```python
from build123d import *

# Parameters (mm, degrees)
SKETCH3_W              = 411.1625
SKETCH3_H              = 277.368
BOSS_EXTRUDE1_DEPTH    = 1.5875
CUT_EXTRUDE1_DEPTH     = 25.4
F_10_CLEARANCE_HOLE1_D = 4.9784
F_10_CLEARANCE_HOLE2_D = 4.9784
F_10_CLEARANCE_HOLE3_D = 4.9784
F_10_CLEARANCE_HOLE4_D = 4.9784
F_10_CLEARANCE_HOLE5_D = 4.9784


with BuildPart() as part:
    # Sketch3 → Boss-Extrude1 (new, symmetric)
    with BuildSketch(Plane.XY):
        Rectangle(SKETCH3_W, SKETCH3_H)
    extrude(amount=BOSS_EXTRUDE1_DEPTH, both=True)

    # Sketch4 → Cut-Extrude1 (cut)
    with BuildSketch(Plane.XY.offset(1.5875)):
        with BuildLine():
            Line((-8.89, 98.4326708), (8.89, 98.4326708))
            ThreePointArc((8.89, 98.4326708), (12.482102448, 96.944773248), (13.97, 93.3526708))
            Line((13.97, 93.3526708), (13.97, 52.7126708))
            ThreePointArc((13.97, 52.7126708), (12.482102448, 49.120568352), (8.89, 47.6326708))
            Line((8.89, 47.6326708), (-8.89, 47.6326708))
            ThreePointArc((-8.89, 47.6326708), (-12.482102448, 49.120568352), (-13.97, 52.7126708))
            Line((-13.97, 52.7126708), (-13.97, 93.3526708))
            ThreePointArc((-13.97, 93.3526708), (-12.482102448, 96.944773248), (-8.89, 98.4326708))
        make_face()
        with BuildLine():
            Line((67.31, 98.4326708), (85.09, 98.4326708))
            ThreePointArc((85.09, 98.4326708), (88.682102448, 96.944773248), (90.17, 93.3526708))
            Line((90.17, 93.3526708), (90.17, 52.7126708))
            ThreePointArc((90.17, 52.7126708), (88.682102448, 49.120568352), (85.09, 47.6326708))
            Line((85.09, 47.6326708), (67.31, 47.6326708))
            ThreePointArc((67.31, 47.6326708), (63.717897552, 49.120568352), (62.23, 52.7126708))
            Line((62.23, 52.7126708), (62.23, 93.3526708))
            ThreePointArc((62.23, 93.3526708), (63.717897552, 96.944773248), (67.31, 98.4326708))
        make_face()
        with BuildLine():
            Line((143.51, 98.4326708), (161.29, 98.4326708))
            ThreePointArc((161.29, 98.4326708), (164.882102448, 96.944773248), (166.37, 93.3526708))
            Line((166.37, 93.3526708), (166.37, 52.7126708))
            ThreePointArc((166.37, 52.7126708), (164.882102448, 49.120568352), (161.29, 47.6326708))
            Line((161.29, 47.6326708), (143.51, 47.6326708))
            ThreePointArc((143.51, 47.6326708), (139.917897552, 49.120568352), (138.43, 52.7126708))
            Line((138.43, 52.7126708), (138.43, 93.3526708))
            ThreePointArc((138.43, 93.3526708), (139.917897552, 96.944773248), (143.51, 98.4326708))
        make_face()
        with BuildLine():
            Line((-85.09, 98.4326708), (-67.31, 98.4326708))
            ThreePointArc((-67.31, 98.4326708), (-63.717897552, 96.944773248), (-62.23, 93.3526708))
            Line((-62.23, 93.3526708), (-62.23, 52.7126708))
            ThreePointArc((-62.23, 52.7126708), (-63.717897552, 49.120568352), (-67.31, 47.6326708))
            Line((-67.31, 47.6326708), (-85.09, 47.6326708))
            ThreePointArc((-85.09, 47.6326708), (-88.682102448, 49.120568352), (-90.17, 52.7126708))
            Line((-90.17, 52.7126708), (-90.17, 93.3526708))
            ThreePointArc((-90.17, 93.3526708), (-88.682102448, 96.944773248), (-85.09, 98.4326708))
        make_face()
        with BuildLine():
            Line((-161.29, 97.1626708), (-146.05, 97.1626708))
            ThreePointArc((-146.05, 97.1626708), (-142.457897552, 95.674773248), (-140.97, 92.0826708))
            Line((-140.97, 92.0826708), (-140.97, 53.9826708))
            ThreePointArc((-140.97, 53.9826708), (-142.457897552, 50.390568352), (-146.05, 48.9026708))
            Line((-146.05, 48.9026708), (-161.29, 48.9026708))
            ThreePointArc((-161.29, 48.9026708), (-164.882102448, 50.390568352), (-166.37, 53.9826708))
            Line((-166.37, 53.9826708), (-166.37, 92.0826708))
            ThreePointArc((-166.37, 92.0826708), (-164.882102448, 95.674773248), (-161.29, 97.1626708))
        make_face()
    extrude(amount=-CUT_EXTRUDE1_DEPTH, mode=Mode.SUBTRACT)

    # #10 Clearance Hole1 (through all)
    with Locations(Plane.XY.offset(1.5875)):
        with Locations((192.88125, 125.984), (-192.88125, -125.984), (192.88125, -125.984), (-192.88125, 125.984), (-192.88125, 0), (192.88125, 0)):
            Hole(F_10_CLEARANCE_HOLE1_D / 2)

    # #10 Clearance Hole2 (through all)
    with Locations(Plane.XY.offset(1.5875)):
        with Locations((0, -117.532545274)):
            Hole(F_10_CLEARANCE_HOLE2_D / 2)

    # #10 Clearance Hole3 (through all)
    with Locations(Plane.XY.offset(1.5875)):
        with Locations((-195.30625, -70.615668917)):
            Hole(F_10_CLEARANCE_HOLE3_D / 2)

    # #10 Clearance Hole4 (through all)
    with Locations(Plane.XY.offset(1.5875)):
        with Locations((-195.30625, -96.015668917)):
            Hole(F_10_CLEARANCE_HOLE4_D / 2)

    # #10 Clearance Hole5 (through all)
    with Locations(Plane.XY.offset(1.5875)):
        with Locations((195.30625, -68.024189157), (195.30625, -93.424189157)):
            Hole(F_10_CLEARANCE_HOLE5_D / 2)


solid = part.part
```
Read the model definition and answer for the solid it produces. Units are mm, in the model's axes. Give positions to 0.01 mm unless a question says otherwise; leave off trailing zeros. Write each loop counter-clockwise with the first axis right and the second up, starting at its lowest first coordinate (ties: lowest second). Pieces come first, ordered by that corner, then holes. Notation, with made-up numbers: M 72.5,42 L 111.5,42 A8 cw 111.5,48 Z; hole C -12.5,87 d8. An arc over 180 degrees is marked long. Put each result on its own line as item: value. Start each with the question number.
1. The part is cut by section B-B, the plane z = 1. Give the number of separate pieces and of enclosed holes in the cut face, and give its area (3 significant figures).
2. This flat-tipped pin is pushed along its axis until it touches: pin 1 Ø3 at (x, y) = (0, -117.53) entering from +Z. Where does it stop, or does it pass through?
3. Consider line 1 along Y through (x, z) = (0, 0.3); line 2 along Y through (x, z) = (6.5, -0.15); line 3 along X through (y, z) = (88, -0.6). Determine where each line is inside the solid, lowest interval first.
4. The part is cut by section A-A, the plane y = 58.5. Give the vertices of the cut face in (x, z).
Final values:
1. separate pieces: 1
1. enclosed holes: 16
1. area: 107,000 mm²
2. pin 1: passes through
3. line 1: y = -138.68 to -120.02, -115.04 to 47.63, 98.43 to 138.68
3. line 2: y = -138.68 to 47.63, 98.43 to 138.68
3. line 3: x = -205.58 to -166.37, -140.97 to -90.17, -62.23 to -13.97, 13.97 to 62.23, 90.17 to 138.43, 166.37 to 205.58
4. outline: M -205.58,-1.59 L -166.37,-1.59 L -166.37,1.59 L -205.58,1.59 Z; M -140.97,-1.59 L -90.17,-1.59 L -90.17,1.59 L -140.97,1.59 Z; M -62.23,-1.59 L -13.97,-1.59 L -13.97,1.59 L -62.23,1.59 Z; M 13.97,-1.59 L 62.23,-1.59 L 62.23,1.59 L 13.97,1.59 Z; M 90.17,-1.59 L 138.43,-1.59 L 138.43,1.59 L 90.17,1.59 Z; M 166.37,-1.59 L 205.58,-1.59 L 205.58,1.59 L 166.37,1.59 Z
